The listing builds one solid part. Answer for the finished solid, in the listing's coordinates (mm). A direction names the side the tool comes from. Round coordinates to 2 decimals unless told otherwise and drop trailing zeros. Write each loop counter-clockwise with the first axis right and the second up, starting at its lowest first coordinate (ties: lowest second). Pieces come first, ordered by that corner, then holes. Notation, with made-up numbers: (15.25, -8.75) - (56.25, -8.75) arc R14 ccw to (56.25, 8.25) - close; hole circle Ø8 at (-34.75, 85). An arc over 180 degrees is marked (long way). Return JSON: item names as keys, results as strings. Group by question number.
from build123d import *

# Parameters (mm, degrees)
CUT_EXTRUDE1_START  = -2.434961
SKETCH2_OUTSIDE_W   = 17.134
SKETCH2_OUTSIDE_H   = 12.156
CUT_EXTRUDE1_DEPTH  = 4.869922
SKETCH7_R           = 2.667
BOSS_EXTRUDE2_DEPTH = 1.51
FILLET1_R           = 0.3
FILLET2_R           = 0.3
FILLET3_R           = 0.3
FILLET4_R           = 0.3


with BuildPart() as part:
    # Sketch1 → Revolve1 (revolve)
    with BuildSketch(Plane(origin=(0, 0, 0), x_dir=(1, 0, 0), z_dir=(0, 1, 0))):
        Polygon((-3.5179, -17.0942), (-1.7272, -17.0942), (-1.7272, -5.6642), (0, -5.6642), (0, -5.08), (-3.5179, -5.08), (-3.5179, -8.382), align=None)
    revolve(axis=Axis((0, 0, 0), (0, 0, 1)))

    # Sketch2 outside → Cut-Extrude1 (cut)
    with BuildSketch(Plane(origin=(0, 0, 0), x_dir=(0, 0, -1), z_dir=(1, 0, 0)).offset(CUT_EXTRUDE1_START)):
        with Locations((-11.087, 0)):
            Rectangle(SKETCH2_OUTSIDE_W, SKETCH2_OUTSIDE_H)
        Polygon((-17.0942, -3.51888695), (-17.0942, 3.51691305), (-13.0302, 3.51691305), (-5.08, 2.53901305), (-5.08, -2.54098695), (-13.0302, -3.51888695), align=None, mode=Mode.SUBTRACT)
    extrude(amount=CUT_EXTRUDE1_DEPTH, mode=Mode.SUBTRACT)

    # Sketch7 → Boss-Extrude2 (add, symmetric)
    with BuildSketch(Plane(origin=(0, 0, 0), x_dir=(1, 0, 0), z_dir=(0, 1, 0))):
        with BuildLine():
            Line((-4.953, 0), (-4.953, -5.08))
            Line((-4.953, -5.08), (-3.5179, -8.382))
            Line((-3.5179, -8.382), (3.5179, -8.382))
            Line((3.5179, -8.382), (4.953, -5.08))
            Line((4.953, -5.08), (4.953, 0))
            ThreePointArc((4.953, 0), (0, 4.953), (-4.953, 0))
        make_face()
        with Locations(Location((0, 0, 0), (0, 0, 90))):
            Circle(SKETCH7_R, mode=Mode.SUBTRACT)
    extrude(amount=BOSS_EXTRUDE2_DEPTH, both=True)

    # Fillet1
    fillet1_edges = [part.edges().sort_by_distance(p)[0] for p in [
        (0, -1.51, -4.953),
        (-4.953, -1.51, 2.54),
        (-4.23545, -1.51, 6.731),
        (4.23545, -1.51, 6.731),
        (4.953, -1.51, 2.54),
    ]]
    fillet(fillet1_edges, radius=FILLET1_R)

    # Fillet2
    fillet2_edges = [part.edges().sort_by_distance(p)[0] for p in [
        (4.23545, 1.51, 6.731),
        (4.953, 1.51, 2.54),
        (0, 1.51, -4.953),
        (-4.953, 1.51, 2.54),
        (-4.23545, 1.51, 6.731),
    ]]
    fillet(fillet2_edges, radius=FILLET2_R)

    # Fillet3
    fillet3_edges = [part.edges().sort_by_distance(p)[0] for p in [
        (0, 1.51, 2.667),
    ]]
    fillet(fillet3_edges, radius=FILLET3_R)

    # Fillet4
    fillet4_edges = [part.edges().sort_by_distance(p)[0] for p in [
        (0, -1.51, 2.667),
    ]]
    fillet(fillet4_edges, radius=FILLET4_R)


solid = part.part
(1) Flat-ended cylindrical pins translate along their axes: pin 1 (0.5 mm diameter, centred on x = 0, z = 7, fed in from -Y); pin 2 (3 mm diameter, centred on x = -2, y = 1, fed in from -Z); pin 3 (0.5 mm diameter, centred on x = -0.5, y = 2, fed in from -Z). Find the tip coordinate at first contact, or state that the pin passes through.
(2) Find section B-B (y = -0.75). Write down the section's boundary in (x, z), plus the area to 3 significant figures.
(3) Find section C-C (z = 6). State how many separate pieces and enclosed holes the cut face has, plus the area to 3 significant figures.
(4) Consider line 1 (X direction, y = 0, z = 12.5); line 2 (Y direction, x = -0.25, z = 13.75); line 3 (Y direction, x = -2.5, z = -2). Determine where each line is inside the solid, lowest interval first.
(5) For faces 5 (the cylindrical face through (-2.36, -2.61, 12.51)), 6 (the flat face through (0, -2, 5.08)), 7 (the flat face through (0, 2, 5.08)), determine the directions among +Z, -Z, +X, -X, +Y, -Y from which every point of the face is accessible in a straight line to the end or side of a thin tool.
(6) Find section A-A (z = 3.25). Write down the section's boundary in (x, y), plus the area to 3 significant figures.
(7) Find section D-D (y = 3). Write down the section's boundary in (x, z).
(8) Determine the mould class of faces 1 (the flat face through (0, 0, 8.382)), 2 (the flat face through (0, -1.51, 7)), 3 (the cylindrical face through (4.14, -1.42, 6.73)), 4 (the cylindrical face through (1.62, -0.02, 2.12)) for opening direction Y: +Y half, -Y half, draft (parallel to the pull), parting line (faces both ways), or undercut.
Check sheet entries:
{
 "1": {"pin 1": "stops at y = -2.81", "pin 2": "stops at z = -4.93", "pin 3": "stops at z = 5.08"},
 "2": {"outline": "(-4.95, 0) arc R4.95 ccw to (4.95, 0) - (4.95, 5.08) - (3.52, 8.38) - (3.44, 8.38) - (3.44, 17.09) - (1.56, 17.09) - (1.56, 8.38) - (-1.56, 8.38) - (-1.56, 17.09) - (-3.44, 17.09) - (-3.44, 8.38) - (-3.52, 8.38) - (-4.95, 5.08) - close; hole circle Ø5.33 at (0, 0)", "area": "127 mm^2"},
 "3": {"separate pieces": "1", "enclosed holes": "2", "area": "39.8 mm^2"},
 "4": {"line 1": "x = -3.52 to -1.73, 1.73 to 3.52", "line 2": "y = -3.51 to -1.71, 1.71 to 3.51", "line 3": "y = -1.51 to 1.51"},
 "5": {"face 5": "+Z", "face 6": "-Z, +X, -X, -Y", "face 7": "-Z, +X, -X, +Y"},
 "6": {"outline": "(-4.95, -1.21) arc R0.3 ccw to (-4.65, -1.51) - (4.65, -1.51) arc R0.3 ccw to (4.95, -1.21) - (4.95, 1.21) arc R0.3 ccw to (4.65, 1.51) - (-4.65, 1.51) arc R0.3 ccw to (-4.95, 1.21) - close", "area": "29.8 mm^2"},
 "7": {"outline": "(-1.84, 8.83) - (1.84, 8.83) - (1.84, 17.09) - (-1.84, 17.09) - close"},
 "8": {"face 1": "undercut", "face 2": "undercut", "face 3": "-Y half", "face 4": "draft"}
}
